```python
from build123d import *

# Parameters (mm, degrees)
F2_SIZE  = 1
F4_DEPTH = 2


with BuildPart() as f1:
    # F0 (on Top) → F1 (revolve)
    with BuildSketch(Plane.XY):
        Polygon((-3, 0), (0, 0), (0, 14.5), (-7.5, 14.5), (-7.5, 12), (-3, 12), align=None)
    revolve(axis=Axis((0, 7.25, 0), (0, -1, 0)))

    # F2
    f2_edges = [f1.edges().sort_by_distance(p)[0] for p in [
        (7.5, 14.5, 0),
        (3, 0, 0),
    ]]
    chamfer(f2_edges, length=F2_SIZE)

    # F3 (on face) → F4 (cut)
    with BuildSketch(Plane(origin=(0, 14.5, 0), x_dir=(-1, 0, 0), z_dir=(0, 1, 0))):
        Polygon((1.154701, 2), (-1.154701, 2), (-2.309401, 0), (-1.154701, -2), (1.154701, -2), (2.309401, 0), align=None)
    extrude(amount=-F4_DEPTH, mode=Mode.SUBTRACT)


solid = f1.part
```
Can you work these out from the model? Positions are in its coordinate system, mm. A direction names the side the tool comes from. Give positions to 0.01 mm unless a question says otherwise; leave off trailing zeros. Loops run counter-clockwise (first coordinate to the right, second up) from the corner with the lowest first, then second, coordinate; pieces in that order, holes last. Notation, with made-up numbers: M 14,-31.5 L 18,-31.5 A18 ccw 18,-22.5 Z; hole C -38,40.5 d3. An arc over 180 degrees is marked long. One line per item, written item: value.
(1) We'd pull the mould along X, two halves only. Please class faces 1 (the face through (0, 0, 0)), 2 (the face through (1.74, 13.51, -0.99)), 3 (the face through (3, 6, 0)): released by +X, released by -X, zero draft, split by the parting line, or undercut.
Returned:
face 1: zero draft
face 2: undercut
face 3: split by the parting line
(2) Will these pins go through, and if not, where does the flat tip stop? pin 1 (8 mm diameter, centred on x = 1, y = 3.5, fed in from +Z); pin 2 (1 mm diameter, centred on y = 13, z = 5, fed in from +X); pin 3 (2 mm diameter, centred on y = 6, z = 0.5, fed in from +X); pin 4 (1.5 mm diameter, centred on y = 8, z = -4.5, fed in from +X).
Returned:
pin 1: z = 3
pin 2: x = 6
pin 3: x = 3
pin 4: through
(3) Suppose I cut it at C-C on y = 6.75. List the corners of the cut face in (x, z) for me.
Returned:
outline: C 0,0 d6
(4) Suppose I cut it at B-B on x = 0. List the corners of the cut face in (y, z) for me, plus the area to 3 significant figures.
Returned:
outline: M 0,-2 L 1,-3 L 12,-3 L 12,-7.5 L 13.5,-7.5 L 14.5,-6.5 L 14.5,-2 L 12.5,-2 L 12.5,2 L 14.5,2 L 14.5,6.5 L 13.5,7.5 L 12,7.5 L 12,3 L 1,3 L 0,2 Z
area: 99.5 mm^2
(5) Suppose I cut it at A-A on y = 13. List the corners of the cut face in (x, z) for me, plus the area to 3 significant figures.
Returned:
outline: C 0,0 d15; hole M -2.31,0 L -1.15,-2 L 1.15,-2 L 2.31,0 L 1.15,2 L -1.15,2 Z
area: 163 mm^2
(6) Which directions (+Z, -Z, +X, -X, +Y, -Y) give clear straight access to the entire face, cutting with the end or side of a thin tool? Please do faces 4 (the face through (-1.724, 13.514, -1.014)), 5 (the face through (-2, 14.5, 1)), 6 (the face through (0.1, 12, 3.2)).
Returned:
face 4: +Y
face 5: +Z, -Z, +X, -X, +Y
face 6: -Y
(7) I need wall thicknesses on line 1 (Y direction, x = 0.5, z = 4); line 2 (Z direction, x = -2.25, y = 14.25); line 3 (Y direction, x = -0.75, z = -1.75). Which ranges of each line are inside material? Lowest first, please.
Returned:
line 1: 12 to 14.5
line 2: -6.36 to -0.1, 0.1 to 6.36
line 3: 0 to 12.5
